Read the model definition and answer for the solid it produces. Units are mm, in the model's axes. A direction names the side the tool comes from. Round coordinates to 2 decimals unless told otherwise and drop trailing zeros. Order: outer loops, then holes, each group sorted by start corner. A loop starts at its lowest first (then second) coordinate and runs counter-clockwise, first axis right, second up.
from build123d import *

# Parameters (mm, degrees)
BOSS_EXTRUDE1_DEPTH     = 20
SKETCH2_R               = 9.3485
BOSS_EXTRUDE2_DEPTH     = 80
FILLET1_R               = 20
CUT_EXTRUDE1_DEPTH      = 126.39936204
CUT_EXTRUDE1_DEPTH_BACK = 126.39936204
SKETCH3_R               = 12.5
SCALE1_SCALE            = 0.5


with BuildPart() as part:
    # Sketch1 → Boss-Extrude1 (new, symmetric)
    with BuildSketch(Plane.XY):
        with BuildLine():
            Line((35, 5), (35, 70))
            ThreePointArc((35, 70), (40, 75), (45, 70))
            Line((45, 70), (45, -5))
            Line((45, -5), (-45, -5))
            Line((-45, -5), (-45, 70))
            ThreePointArc((-45, 70), (-40, 75), (-35, 70))
            Line((-35, 70), (-35, 5))
            Line((-35, 5), (35, 5))
        make_face()
    extrude(amount=BOSS_EXTRUDE1_DEPTH, both=True)

    # Sketch2 → Boss-Extrude2 (add)
    with BuildSketch(Plane.XZ.offset(5)):
        with Locations(Location((0, 0, 0), (0, 0, 270))):
            Circle(SKETCH2_R)
    extrude(amount=BOSS_EXTRUDE2_DEPTH)

    # Fillet1
    fillet1_edges = [part.edges().sort_by_distance(p)[0] for p in [
        (35, 5, 0),
        (45, -5, 0),
        (-45, -5, 0),
        (-35, 5, 0),
    ]]
    fillet(fillet1_edges, radius=FILLET1_R)

    # Sketch3 → Cut-Extrude1 (cut, two sides: drawn at the far end of the back side and taken through both)
    with BuildSketch(Plane(origin=(45, 0, 0), x_dir=(0, 0, -1), z_dir=(1, 0, 0)).offset(-CUT_EXTRUDE1_DEPTH_BACK)):
        with Locations(Location((0, 55, 0), (0, 0, 90))):
            Circle(SKETCH3_R)
    extrude(amount=CUT_EXTRUDE1_DEPTH + CUT_EXTRUDE1_DEPTH_BACK, mode=Mode.SUBTRACT)


with BuildPart() as part_1:
    # Scale1: scaled about (0, 6.940558609, 0)
    add(part.part.scale(SCALE1_SCALE).moved(Location((0, 3.470279304, 0))))


solid = part_1.part
Q1. Flat-ended cylindrical pins translate along their axes: pin 1 (8 mm diameter, centred on x = -17.5, y = -1, fed in from +Z); pin 2 (8 mm diameter, centred on x = -1, z = 7, fed in from +Y); pin 3 (8 mm diameter, centred on y = -29.5, z = -6, fed in from +X); pin 4 (1 mm diameter, centred on x = 10.5, z = 3, fed in from -Y). Find the tip coordinate at first contact, or state that the pin passes through.
Outcome:
pin 1: stops at z = 10
pin 2: stops at y = 5.97
pin 3: stops at x = 4.22
pin 4: stops at y = 0.97
Q2. A cutting plane is placed at D-D, the plane z = -8.25. Give the vertices of the cut face in (x, y).
Outcome:
outline: (-22.5, 10.97) arc R10 ccw to (-12.5, 0.97) - (12.5, 0.97) arc R10 ccw to (22.5, 10.97) - (22.5, 38.47) arc R2.5 ccw to (17.5, 38.47) - (17.5, 15.97) arc R10 cw to (7.5, 5.97) - (-7.5, 5.97) arc R10 cw to (-17.5, 15.97) - (-17.5, 38.47) arc R2.5 ccw to (-22.5, 38.47) - close
Q3. A cutting plane is placed at B-B, the plane x = 0. Give the vertices of the cut face in (y, z).
Outcome:
outline: (-39.03, -4.67) - (0.97, -4.67) - (0.97, -10) - (5.97, -10) - (5.97, 10) - (0.97, 10) - (0.97, 4.67) - (-39.03, 4.67) - close
Q4. A cutting plane is placed at A-A, the plane z = 0. Give the vertices of the cut face in (x, y).
Outcome:
outline: (-22.5, 10.97) arc R10 ccw to (-12.5, 0.97) - (-4.67, 0.97) - (-4.67, -39.03) - (4.67, -39.03) - (4.67, 0.97) - (12.5, 0.97) arc R10 ccw to (22.5, 10.97) - (22.5, 24.72) - (17.5, 24.72) - (17.5, 15.97) arc R10 cw to (7.5, 5.97) - (-7.5, 5.97) arc R10 cw to (-17.5, 15.97) - (-17.5, 24.72) - (-22.5, 24.72) - close; (-22.5, 37.22) - (-17.5, 37.22) - (-17.5, 38.47) arc R2.5 ccw to (-22.5, 38.47) - close; (17.5, 37.22) - (22.5, 37.22) - (22.5, 38.47) arc R2.5 ccw to (17.5, 38.47) - close
Q5. For faces 1 (the face through (2, 5, 10)), 2 (the face through (3.159, -18.75, 3.445)), 3 (the face through (-14.49, 8.82, 0.14)), determine the directions among +Z, -Z, +X, -X, +Y, -Y from which every point of the face is accessible in a straight line to the end or side of a thin tool.
Outcome:
face 1: +Z, +X, -X, +Y, -Y
face 2: -Y
face 3: +Z, -Z, +Y
Q6. A cutting plane is placed at C-C, the plane y = 25.5. Give the vertices of the cut face in (x, z), plus the area to 3 significant figures.
Outcome:
outline: (-22.5, -10) - (-17.5, -10) - (-17.5, -3.02) - (-22.5, -3.02) - close; (-22.5, 3.02) - (-17.5, 3.02) - (-17.5, 10) - (-22.5, 10) - close; (17.5, -10) - (22.5, -10) - (22.5, -3.02) - (17.5, -3.02) - close; (17.5, 3.02) - (22.5, 3.02) - (22.5, 10) - (17.5, 10) - close
area: 140 mm2
Q7. Straight lines are drawn through the part: probe 1 along X at (y, z) = (29.5, -6.5); probe 2 along Z at (x, y) = (-18, 31); probe 3 along Y at (x, z) = (20.2, 0). For each, find the intervals that lie inside material, in ascending order.
Outcome:
probe 1: x = -22.5 to -17.5, 17.5 to 22.5
probe 2: z = -10 to -6.25, 6.25 to 10
probe 3: y = 4.59 to 24.72, 37.22 to 40.96
Q8. For a pull along X with two mould halves and no side action, classify faces 4 (the face through (19.65, 3.98, -0.14)), 5 (the face through (-3, 0.97, 5)), 6 (the face through (-19.49, 3.82, -0.14)), 7 (the face through (-20.05, 40.97, 0.14)) as released by +X, released by -X, zero draft, split by the parting line, or undercut.
Outcome:
face 4: released by +X
face 5: zero draft
face 6: released by -X
face 7: undercut
